Job drawing, mm, ordinate dimensions from the low corner. One solid piece. A direction names the side the tool comes from. Round coordinates to 2 decimals unless told otherwise and drop trailing zeros. Write each loop counter-clockwise with the first axis right and the second up, starting at its lowest first coordinate (ties: lowest second). Pieces come first, ordered by that corner, then holes.
1) Wall check: probe 1 along Y at (x, z) = (5, 11.25); probe 2 along X at (y, z) = (25.5, 4.5) (1 decimal); probe 3 along Z at (x, y) = (2.25, 16.5) (1 decimal). Give the ranges that are in metal, low to high.
2) Saw through at C-C (x = 1). Write the cut outline in (y, z), plus the area to 3 significant figures.
3) Flat gauge pins, fed straight in: pin 1 (1.5 mm diameter, centred on x = 2.5, y = 35.5, fed in from +Z); pin 2 (6 mm diameter, centred on y = 34.5, z = 5.5, fed in from +X); pin 3 (1.5 mm diameter, centred on x = 5, y = 23.5, fed in from +Z). Where does each tip first touch, or does it go through?
4) Saw through at D-D (y = 15). Write the cut outline in (x, z).
5) Saw through at A-A (y = 3.5). Write the cut outline in (x, z), plus the area to 3 significant figures.
6) Which spindle directions (+Z, -Z, +X, -X, +Y, -Y) get a long thin tool onto all of the face, cutting with end or side? Do the marked faces 1 and 2. Say none if no direction does.
7) Saw through at B-B (z = 9.75). Write the cut outline in (x, y), plus the area to 3 significant figures.
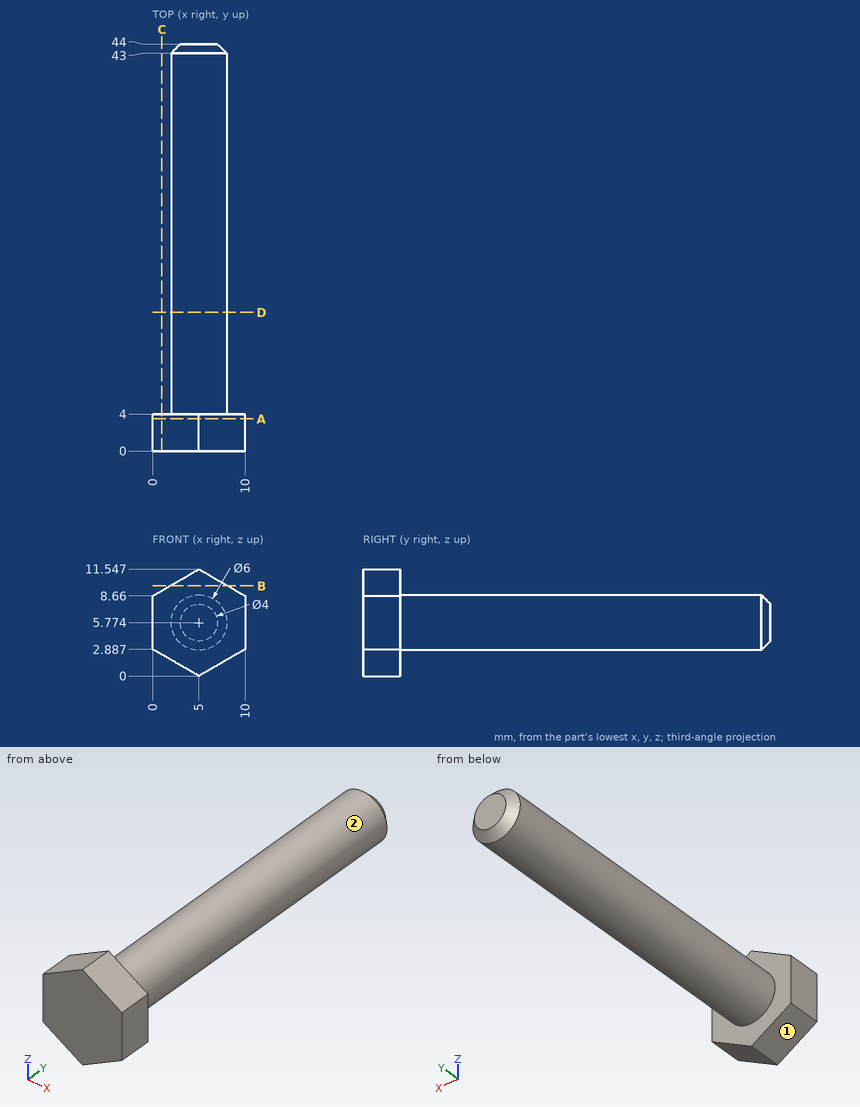
Evaluation:
1. probe 1: y = 0 to 4
1. probe 2: x = 2.3 to 7.7
1. probe 3: z = 4.6 to 7
2. outline: (0, 2.31) - (4, 2.31) - (4, 9.24) - (0, 9.24) - close
2. area: 27.7 mm2
3. pin 1: stops at z = 8.21
3. pin 2: stops at x = 8
3. pin 3: stops at z = 8.77
4. outline: circle Ø6 at (5, 5.77)
5. outline: (0, 2.89) - (5, 0) - (10, 2.89) - (10, 8.66) - (5, 11.55) - (0, 8.66) - close
5. area: 86.6 mm2
6. face 1: -Z, -X, +Y, -Y
6. face 2: +Y
7. outline: (1.89, 0) - (8.11, 0) - (8.11, 4) - (1.89, 4) - close
7. area: 24.9 mm2
